Check sheet for the modelled part. Datum: model origin and axes. Units: mm. Face numbers are marked on the shaded views. Give positions to 0.01 mm unless a question says otherwise; leave off trailing zeros. Loops run counter-clockwise (first coordinate to the right, second up) from the corner with the lowest first, then second, coordinate; pieces in that order, holes last. Notation, with made-up numbers: (64, -9) - (73, -9) arc R25 cw to (73, 18) - close; hole circle Ø8 at (88.25, 62). An arc over 180 degrees is marked (long way). Answer in a Markdown table with one row per item. Add a question column.
(1) Sectioned sample at B-B on z = 28.2. Enter the section's corners in (x, y).
(2) Draft check along Z on the marked faces 1, 2 and 3. Enter one of: released by +Z, released by -Z, zero draft, split by the parting line, or undercut.
(3) Sectioned sample at A-A on y = -5. Enter the section's corners in (x, z), then the cut area to 3 significant figures.
(4) Sectioned sample at C-C on x = 12.25. Enter the section's corners in (y, z), then the cut area to 3 significant figures.
(5) Sectioned sample at D-D on y = -7.75. Enter the section's corners in (x, z).
(6) Go/stop test with flat-tipped pins: P1, Ø5, axis at x = 19, y = -6, coming from the +Z side; P2, Ø1, axis at y = -4, z = 28, coming from the -X side. Record where each tip stops, or that it passes through.
(7) Thickness scan on L1, parallel to X at y = -6, z = 26.2; L2, parallel to X at y = -5, z = 28.9; L3, parallel to Z at x = 17.75, y = -7.5. Record the ranges inside material, lowest first.
from build123d import *

# Parameters (mm, degrees)
F1_DEPTH = 10
F3_D     = 3


# Not quite as in the source:
# - ends of sketch curves that miss each other by under 0.0002 mm in the source are joined


with BuildPart() as f1:
    # F0 (on Front) → F1 (new body)
    with BuildSketch(Plane.XZ):
        with BuildLine():
            ThreePointArc((13.5271953943, 27.6566442743), (9.210189973, 31.473808666), (10.8152050392, 25.9392620325))
            Line((10.8152050392, 25.9392620325), (30.8152050392, 25.9392620325))
            Line((30.8152050392, 25.9392620325), (30.8152050392, 26.439262554))
            Line((30.8152050392, 26.439262554), (10.8152050392, 26.439262554))
            ThreePointArc((10.8152050392, 26.439262554), (9.4776924841, 31.0513842271), (13.0751970018, 27.8704139006))
            Line((13.0751970018, 27.8704139006), (13.5271953943, 27.6566442743))
        make_face()
    extrude(amount=F1_DEPTH)

    # F3 (through all)
    with Locations(Plane.XY.offset(26.439262554)):
        with Locations((16.4454622901, -5), (25.1849477884, -5)):
            Hole(F3_D / 2)


solid = f1.part
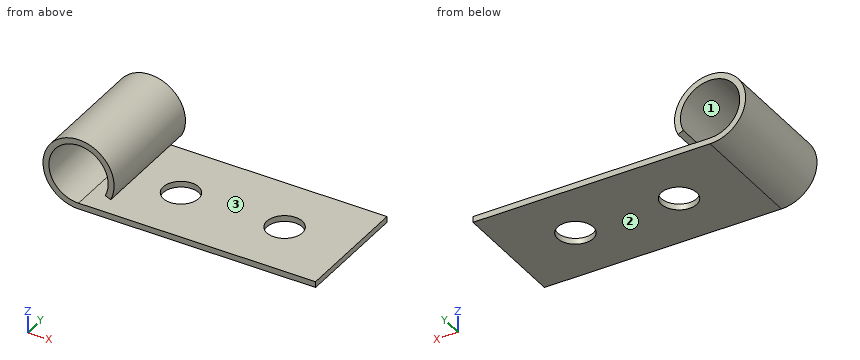
Reply:
| question | item | result |
|---|---|---|
| 1 | outline | (7.91, -10) - (8.43, -10) - (8.43, 0) - (7.91, 0) - close; (13.2, -10) - (13.72, -10) - (13.72, 0) - (13.2, 0) - close |
| 2 | face 1 | undercut |
| 2 | face 2 | released by -Z |
| 2 | face 3 | undercut |
| 3 | outline | (10.82, 25.94) - (14.95, 25.94) - (14.95, 26.44) - (10.82, 26.44) arc R2.5 cw (long way) to (13.08, 27.87) - (13.53, 27.66) arc R3 ccw (long way) to start; (17.95, 25.94) - (23.68, 25.94) - (23.68, 26.44) - (17.95, 26.44) - close; (26.68, 25.94) - (30.82, 25.94) - (30.82, 26.44) - (26.68, 26.44) - close |
| 3 | area | 14.1 mm^2 |
| 4 | outline | (-10, 25.94) - (0, 25.94) - (0, 26.44) - (-10, 26.44) - close; (-10, 30.99) - (0, 30.99) - (0, 31.57) - (-10, 31.57) - close |
| 4 | area | 10.9 mm^2 |
| 5 | outline | (10.82, 25.94) - (30.82, 25.94) - (30.82, 26.44) - (10.82, 26.44) arc R2.5 cw (long way) to (13.08, 27.87) - (13.53, 27.66) arc R3 ccw (long way) to start |
| 6 | P1 | z = 26.44 |
| 6 | P2 | x = 7.85 |
| 7 | L1 | 9.59 to 15.33, 17.56 to 24.07, 26.3 to 30.82 |
| 7 | L2 | 7.82 to 8.32, 13.31 to 13.81 |
| 7 | L3 | 25.94 to 26.44 |
